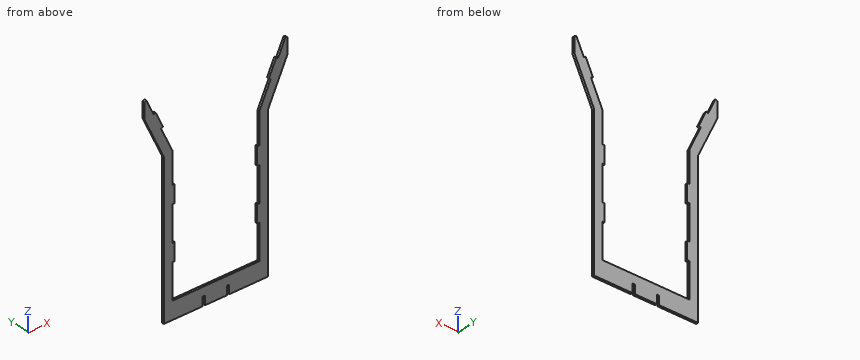
from build123d import *

# Parameters (mm, degrees)
BASE_FLANGE1_DEPTH = 3.175
SKETCH7_W          = 3.175
SKETCH7_H          = 12.7
CUT_EXTRUDE1_DEPTH = 326.126156068
SKETCH12_W         = 3.175
SKETCH12_H         = 25.4
TAB1_DEPTH         = 3.175
CUT_EXTRUDE2_DEPTH = 326.126156068


# Sheet-metal steps are written as plain solids
with BuildPart() as part:
    # Sketch1 → Base-Flange1 (new body)
    with BuildSketch(Plane(origin=(0, 0, 0), x_dir=(1, 0, 0), z_dir=(0, 1, 0))):
        Polygon((-76.2, 0), (76.2, 0), (76.2, -220.278764113), (113.110108895, -299.432748076), (101.6, -304.8), (63.5, -223.094286329), (63.5, -25.4), (-63.5, -25.4), (-63.5, -223.094286329), (-101.6, -304.8), (-113.110108895, -299.432748076), (-76.2, -220.278764113), align=None)
    extrude(amount=-BASE_FLANGE1_DEPTH)

    # Sketch7 → Cut-Extrude1 (cut, through all)
    with BuildSketch(Plane(origin=(0, 0, 0), x_dir=(1, 0, 0), z_dir=(0, 1, 0))):
        with Locations((-17.7165, -6.35)):
            Rectangle(SKETCH7_W, SKETCH7_H)
        with Locations((17.7165, -6.35)):
            Rectangle(SKETCH7_W, SKETCH7_H)
    extrude(amount=-CUT_EXTRUDE1_DEPTH, mode=Mode.SUBTRACT)

    # Sketch12 → Tab1 (add)
    with BuildSketch(Plane(origin=(0, 0, 0), x_dir=(1, 0, 0), z_dir=(0, 1, 0))):
        with Locations((-61.9125, -88.9)):
            Rectangle(SKETCH12_W, SKETCH12_H)
        Polygon((-80.130992304, -258.759564419), (-90.865496152, -281.779782209), (-87.987968928, -283.12159519), (-77.25346508, -260.1013774), align=None)
        with Locations((-61.9125, -165.1)):
            Rectangle(SKETCH12_W, SKETCH12_H)
        Polygon((77.25346508, -260.1013774), (87.987968928, -283.12159519), (90.865496152, -281.779782209), (80.130992304, -258.759564419), align=None)
        with Locations((61.9125, -165.1)):
            Rectangle(SKETCH12_W, SKETCH12_H)
        with Locations((61.9125, -88.9)):
            Rectangle(SKETCH12_W, SKETCH12_H)
    extrude(amount=-TAB1_DEPTH)

    # Sketch13 → Cut-Extrude2 (cut, through all)
    with BuildSketch(Plane(origin=(0, 0, 0), x_dir=(1, 0, 0), z_dir=(0, 1, 0))):
        Polygon((-104.477527224, -303.458187019), (-104.477527224, -280.920116939), (-113.110108895, -299.432748076), align=None)
        Polygon((104.477527224, -303.458187019), (104.477527224, -280.920116939), (113.110108895, -299.432748076), align=None)
    extrude(amount=-CUT_EXTRUDE2_DEPTH, mode=Mode.SUBTRACT)


solid = part.part
For this review, take the finished solid that the model builds, in its own axes (mm). Give positions to 0.01 mm unless a question says otherwise; leave off trailing zeros. Order: outer loops, then holes, each group sorted by start corner. A loop starts at its lowest first (then second) coordinate and runs counter-clockwise, first axis right, second up. Notation, with made-up numbers: (60, -17.5) - (102, -17.5) arc R21 ccw to (102, -11.5) - close; hole circle Ø7 at (4.5, 58). An arc over 180 degrees is marked (long way). Answer as a JSON object with one key per item and string values. Group by question number.
Item 1: Clearance check with flat-ended pins moving along their axes: pin 1 Ø1.6 at (y, z) = (-2.5, 119.5) entering from +X; pin 2 Ø1.5 at (x, y) = (72, -1.5) entering from +Z; pin 3 Ø10 at (x, z) = (54.5, 150) entering from +Y; pin 4 Ø1.5 at (x, y) = (38.5, -2.5) entering from +Z. State where each tip first meets the part, or that it passes through.
Item 2: Take a section at B-B on x = 36.5. Give the boundary of the cut face in (y, z) (3 decimals).
Item 3: Take a section at D-D on x = -67. Give the boundary of the cut face in (y, z) (3 decimals).
Item 4: Take a section at C-C on z = 239. Give the boundary of the cut face in (x, y) (3 decimals), and give its area (3 significant figures).
Item 5: Take a section at A-A on z = 159.5. Give the boundary of the cut face in (x, y) (3 decimals), and give its area (3 significant figures).
Item 6: Wall thickness on line 1 along X through (y, z) = (-0.2, 178); line 2 along X through (y, z) = (-2.1, 79) (3 decimals); line 3 along Z through (x, y) = (-35, -2.2): over which ranges is each line inside the solid? List them lowest first.
Reported:
{
 "1": {"pin 1": "x = 76.2", "pin 2": "z = 242.93", "pin 3": "through", "pin 4": "z = 25.4"},
 "2": {"outline": "(-3.175, 0) - (0, 0) - (0, 25.4) - (-3.175, 25.4) - close"},
 "3": {"outline": "(-3.175, 0) - (0, 0) - (0, 230.6) - (-3.175, 230.6) - close"},
 "4": {"outline": "(-84.93, -3.175) - (-70.917, -3.175) - (-70.917, 0) - (-84.93, 0) - close; (70.917, -3.175) - (84.93, -3.175) - (84.93, 0) - (70.917, 0) - close", "area": "89.0 mm^2"},
 "5": {"outline": "(-76.2, -3.175) - (-60.325, -3.175) - (-60.325, 0) - (-76.2, 0) - close; (60.325, -3.175) - (76.2, -3.175) - (76.2, 0) - (60.325, 0) - close", "area": "101 mm^2"},
 "6": {"line 1": "-76.2 to -63.5, 63.5 to 76.2", "line 2": "-76.2 to -60.325, 60.325 to 76.2", "line 3": "0 to 25.4"}
}
